Input: part model. Units: mm. Frame: model coordinates. Round coordinates to 2 decimals unless told otherwise and drop trailing zeros. Write each loop counter-clockwise with the first axis right and the second up, starting at its lowest first coordinate (ties: lowest second). Pieces come first, ordered by that corner, then holes. Notation, with made-up numbers: (79, 25.25) - (133, 25.25) arc R30 ccw to (133, 62.25) - close; hole circle Ø4 at (-28, 83). An arc over 180 degrees is marked (long way). One line per item, written item: value. Start each with the question number.
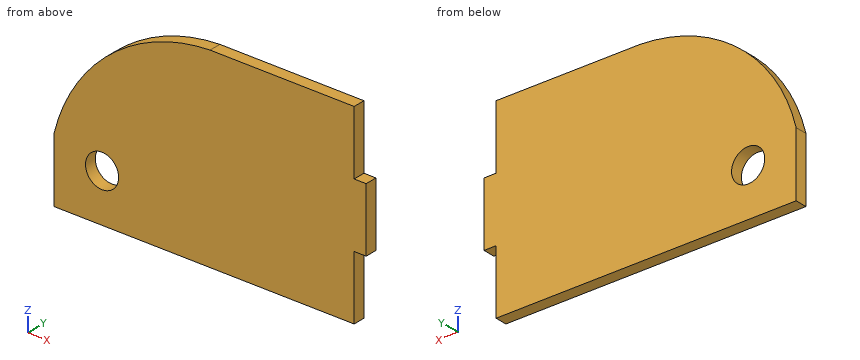
```python
from build123d import *

# Parameters (mm, degrees)
F0_W     = 82.55
F0_H     = 50.8
F1_DEPTH = 3.175
F2_R     = 4.3815
F3_DEPTH = 3.175
F5_DEPTH = 3.175
F6_W     = 3.175
F6_H     = 16.9333333333
F7_DEPTH = 3.175


with BuildPart() as f1:
    # F0 (on Front) → F1 (new body)
    with BuildSketch(Plane.XZ):
        Rectangle(F0_W, F0_H)
    extrude(amount=F1_DEPTH)

    # F2 (on face) → F3 (cut)
    with BuildSketch(Plane.XZ.offset(3.175)):
        with Locations((-28.575, -12.7)):
            Circle(F2_R)
    extrude(amount=-F3_DEPTH, mode=Mode.SUBTRACT)

    # F4 (on face) → F5 (cut)
    with BuildSketch(Plane.XZ.offset(3.175)):
        with BuildLine():
            ThreePointArc((-41.275, -8.3196220329), (-26.2518600879, 15.4125291421), (0, 25.4))
            Line((0, 25.4), (-41.275, 25.4))
            Line((-41.275, 25.4), (-41.275, -8.3196220329))
        make_face()
    extrude(amount=-F5_DEPTH, mode=Mode.SUBTRACT)

    # F6 (on face) → F7 (cut)
    with BuildSketch(Plane.XZ.offset(3.175)):
        with Locations((39.6875, 16.9333333333)):
            Rectangle(F6_W, F6_H)
        with Locations((39.6875, -16.9333333333)):
            Rectangle(F6_W, F6_H)
    extrude(amount=-F7_DEPTH, mode=Mode.SUBTRACT)


solid = f1.part
```
Q1. Cut plane A-A, the plane z = -12.7. Output: boundary loops of the cut face in (x, y) (1 decimal).
Q2. Cut plane B-B, the plane x = -32. Output: boundary loops of the cut face in (y, z) (3 decimals).
Q3. Material intervals for probe 1 along X at (y, z) = (-2, -13) (3 decimals); probe 2 along X at (y, z) = (-0.65, 17); probe 3 along X at (y, z) = (-2.65, -15) (3 decimals), sorted ascending. Write a range as from..to.
Q4. Cut plane D-D, the plane z = 19.5. Output: boundary loops of the cut face in (x, y) (3 decimals), and give its area (3 significant figures).
Q5. Contact query for flat-ended pins moving along their axis: pin 1 Ø5.5 at (x, z) = (-28.575, -12.7) entering from +Y; pin 2 Ø1.5 at (x, y) = (-30.5, -1) entering from +Z; pin 3 Ø1 at (x, y) = (-9, -2.5) entering from +Z. Output: stop coordinate, or through.
A:
1. outline: (-41.3, -3.2) - (-33, -3.2) - (-33, 0) - (-41.3, 0) - close; (-24.2, -3.2) - (38.1, -3.2) - (38.1, 0) - (-24.2, 0) - close
2. outline: (-3.175, -25.4) - (0, -25.4) - (0, -15.433) - (-3.175, -15.433) - close; (-3.175, -9.967) - (0, -9.967) - (0, 9.775) - (-3.175, 9.775) - close
3. probe 1: x = -41.275..-32.946, -24.204..38.1
3. probe 2: x = -24.19..38.1
3. probe 3: x = -41.275..-32.304, -24.846..38.1
4. outline: (-20.327, -3.175) - (38.1, -3.175) - (38.1, 0) - (-20.327, 0) - close
4. area: 186 mm²
5. pin 1: passes through
5. pin 2: stops at z = 12.23
5. pin 3: stops at z = 24.21
